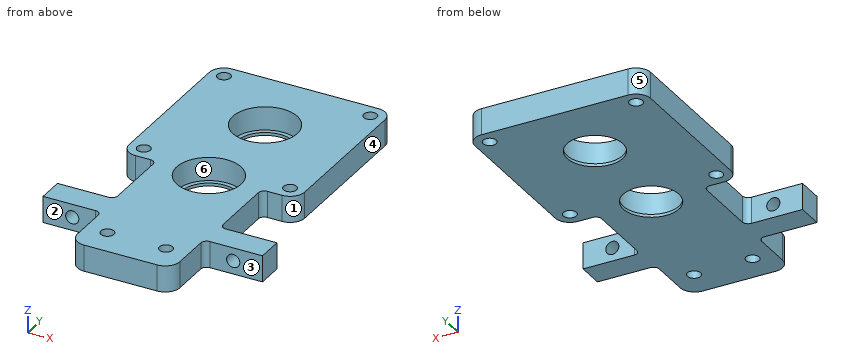
```python
from build123d import *

# Parameters (mm, degrees)
ESQUISSE1_W                  = 75
ESQUISSE1_H                  = 95
BOSS_EXTRU_1_DEPTH           = 9
ESQUISSE2_W                  = 35
ESQUISSE2_H                  = 20
BOSS_EXTRU_2_DEPTH           = 9
ESQUISSE3_R                  = 11
ENL_V_MAT_EXTRU_1_DEPTH      = 8
ESQUISSE4_R                  = 9.5
ENL_V_MAT_EXTRU_2_DEPTH      = 122.371331047
ENL_V_MAT_EXTRU_3_DEPTH      = 122.371331047
ENL_V_MAT_EXTRU_3_DEPTH_BACK = 122.371331047
ESQUISSE5_W                  = 7.5
ESQUISSE5_H                  = 86
ENL_V_START                  = -9
ESQUISSE8_W                  = 12
ESQUISSE8_H                  = 26
ENL_V_MAT_EXTRU_6_DEPTH      = 9
CONG_1_R                     = 2
CONG_2_R                     = 5
ESQUISSE6_R                  = 2.25
ENL_V_MAT_EXTRU_4_DEPTH      = 122.371331047
ESQUISSE7_R                  = 2.25
ENL_V_MAT_EXTRU_5_DEPTH      = 115.46396813


with BuildPart() as part:
    # Esquisse1 → Boss.-Extru.1 (new body)
    with BuildSketch(Plane.XY):
        with Locations((37.5, 47.5)):
            Rectangle(ESQUISSE1_W, ESQUISSE1_H)
    extrude(amount=BOSS_EXTRU_1_DEPTH)

    # Esquisse2 → Boss.-Extru.2 (add)
    with BuildSketch(Plane.XY.offset(9)):
        with Locations((37.5, -10)):
            Rectangle(ESQUISSE2_W, ESQUISSE2_H)
    extrude(amount=-BOSS_EXTRU_2_DEPTH)

    # Esquisse3 → Enlèv. mat.-Extru.1 (cut)
    with BuildSketch(Plane.XY.offset(9)):
        with Locations((37.5, 70)):
            Circle(ESQUISSE3_R)
        with Locations((37.5, 35)):
            Circle(ESQUISSE3_R)
    extrude(amount=-ENL_V_MAT_EXTRU_1_DEPTH, mode=Mode.SUBTRACT)

    # Esquisse4 → Enlèv. mat.-Extru.2 (cut, through all)
    with BuildSketch(Plane.XY.offset(9)):
        with Locations((37.5, 70)):
            Circle(ESQUISSE4_R)
        with Locations((37.5, 35)):
            Circle(ESQUISSE4_R)
    extrude(amount=-ENL_V_MAT_EXTRU_2_DEPTH, mode=Mode.SUBTRACT)

    # Esquisse5 → Enlèv. mat.-Extru.3 (cut, two sides: drawn at the far end of the back side and taken through both)
    with BuildSketch(Plane.XY.offset(9).offset(-ENL_V_MAT_EXTRU_3_DEPTH_BACK)):
        with Locations((71.25, 52)):
            Rectangle(ESQUISSE5_W, ESQUISSE5_H)
        with Locations((3.75, 52)):
            Rectangle(ESQUISSE5_W, ESQUISSE5_H)
    extrude(amount=ENL_V_MAT_EXTRU_3_DEPTH + ENL_V_MAT_EXTRU_3_DEPTH_BACK, mode=Mode.SUBTRACT)

    # Esquisse8 → Enlèv. mat.-Extru.6 (cut)
    with BuildSketch(Plane.XY.offset(9).offset(ENL_V_START)):
        with Locations((13.5, 22)):
            Rectangle(ESQUISSE8_W, ESQUISSE8_H)
        with Locations((61.5, 22)):
            Rectangle(ESQUISSE8_W, ESQUISSE8_H)
    extrude(amount=ENL_V_MAT_EXTRU_6_DEPTH, mode=Mode.SUBTRACT)

    # Congé1
    cong_1_edges = [part.edges().sort_by_distance(p)[0] for p in [
        (55.5, 9, 4.5),
        (55.5, 35, 4.5),
        (20, 0, 4.5),
        (55, 0, 4.5),
        (19.5, 35, 4.5),
        (19.5, 9, 4.5),
    ]]
    fillet(cong_1_edges, radius=CONG_1_R)

    # Congé2
    cong_2_edges = [part.edges().sort_by_distance(p)[0] for p in [
        (67.5, 35, 4.5),
        (20, -20, 4.5),
        (55, -20, 4.5),
        (67.5, 95, 4.5),
        (7.5, 95, 4.5),
        (7.5, 35, 4.5),
    ]]
    fillet(cong_2_edges, radius=CONG_2_R)

    # Esquisse6 → Enlèv. mat.-Extru.4 (cut, through all)
    with BuildSketch(Plane.XY.offset(9)):
        with Locations((47.5, -10)):
            Circle(ESQUISSE6_R)
        with Locations(Location((27.5, -10, 0), (0, 0, 180))):
            Circle(ESQUISSE6_R)
        with Locations((12.5, 90)):
            Circle(ESQUISSE6_R)
        with Locations((12.5, 40)):
            Circle(ESQUISSE6_R)
        with Locations(Location((62.5, 40, 0), (0, 0, 180))):
            Circle(ESQUISSE6_R)
        with Locations(Location((62.5, 90, 0), (0, 0, 180))):
            Circle(ESQUISSE6_R)
    extrude(amount=-ENL_V_MAT_EXTRU_4_DEPTH, mode=Mode.SUBTRACT)

    # Esquisse7 → Enlèv. mat.-Extru.5 (cut, through all)
    with BuildSketch(Plane(origin=(0, 9, 0), x_dir=(1, 0, 0), z_dir=(0, 1, 0))):
        with Locations(Location((10, -4.5, 0), (0, 0, 180))):
            Circle(ESQUISSE7_R)
        with Locations(Location((65, -4.5, 0), (0, 0, 270))):
            Circle(ESQUISSE7_R)
    extrude(amount=-ENL_V_MAT_EXTRU_5_DEPTH, mode=Mode.SUBTRACT)


solid = part.part
```
The listing builds one solid part. Answer for the finished solid, in the listing's coordinates (mm). Face numbers are marked on the shaded views. A direction names the side the tool comes from. Give positions to 0.01 mm unless a question says otherwise; leave off trailing zeros. Loops run counter-clockwise (first coordinate to the right, second up) from the corner with the lowest first, then second, coordinate; pieces in that order, holes last. Notation, with made-up numbers: M 62,4.5 L 96,4.5 A21 cw 96,23.5 Z; hole C -1,80 d10. An arc over 180 degrees is marked long. One line per item, written item: value.
1. For the marked faces 1, 2 and 3, determine the directions among +Z, -Z, +X, -X, +Y, -Y from which every point of the face is accessible in a straight line to the end or side of a thin tool.
Found:
face 1: +Z, -Z, +X
face 2: +Z, -Z, -X, -Y
face 3: +Z, -Z, +X, -Y
2. Each of these flat-tipped pins is pushed along its axis until it touches: P1, Ø2.5, axis at y = 22, z = 3, coming from the -X side; P2, Ø4, axis at x = 52.5, z = 4, coming from the -Y side; P3, Ø4.5, axis at y = 54, z = 5.5, coming from the -X side. Where does it stop, or does it pass through?
Found:
P1: x = 19.5
P2: y = -19.97
P3: x = 7.5
3. Section C-C on y = 4.5 is taken. Determine the outline of the cut face in (x, z).
Found:
outline: M 0,0 L 75,0 L 75,9 L 0,9 Z; hole C 10,4.5 d4.5; hole C 65,4.5 d4.5
4. Section B-B on x = 36 is taken. Determine the outline of the cut face in (y, z), plus the area to 3 significant figures.
Found:
outline: M -20,0 L 25.62,0 L 25.62,1 L 24.1,1 L 24.1,9 L -20,9 Z; M 44.38,0 L 60.62,0 L 60.62,1 L 59.1,1 L 59.1,9 L 45.9,9 L 45.9,1 L 44.38,1 Z; M 79.38,0 L 95,0 L 95,9 L 80.9,9 L 80.9,1 L 79.38,1 Z
area: 649 mm^2
5. Find the intervals of material crossed by probe 1 along Y at (x, z) = (37.5, 4); probe 2 along Y at (x, z) = (12.5, 4); probe 3 along Y at (x, z) = (29.5, 4), in increasing order.
Found:
probe 1: -20 to 24, 46 to 59, 81 to 95
probe 2: 0 to 9, 35 to 37.75, 42.25 to 87.75, 92.25 to 95
probe 3: -20 to -11.03, -8.97 to 27.45, 42.55 to 62.45, 77.55 to 95
6. Section A-A on y = 70 is taken. Determine the outline of the cut face in (x, z).
Found:
outline: M 7.5,0 L 28,0 L 28,1 L 26.5,1 L 26.5,9 L 7.5,9 Z; M 47,0 L 67.5,0 L 67.5,9 L 48.5,9 L 48.5,1 L 47,1 Z
7. Section D-D on y = 28 is taken. Determine the outline of the cut face in (x, z), plus the area to 3 significant figures.
Found:
outline: M 19.5,0 L 31.08,0 L 31.08,1 L 29.01,1 L 29.01,9 L 19.5,9 Z; M 43.92,0 L 55.5,0 L 55.5,9 L 45.99,9 L 45.99,1 L 43.92,1 Z
area: 175 mm^2
8. For a pull along X with two mould halves and no side action, classify the marked faces 4, 5 and 6 as pulls with the +X half, pulls with the -X half, needs draft (parallel to the pull), parting line crosses it, or undercut.
Found:
face 4: pulls with the +X half
face 5: pulls with the -X half
face 6: undercut
